from build123d import *

# Parameters (mm, degrees)
F1_DEPTH = 50


with BuildPart() as f1:
    # F0 (on Right) → F1 (new body)
    with BuildSketch(Plane.YZ):
        Polygon((40, 40), (0, 0), (4.242641, 0), (12, 7.757359), (44.242641, 40), align=None)
        Polygon((12, 7.757359), (4.242641, 0), (12, 0), align=None)
    extrude(amount=F1_DEPTH)


solid = f1.part
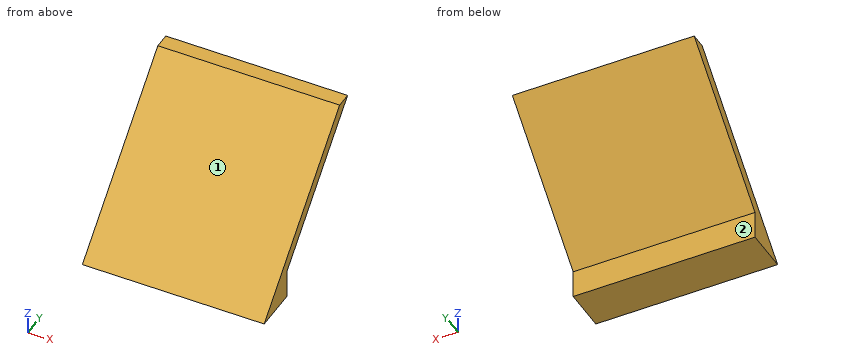
The listing builds one solid part. Answer for the finished solid, in the listing's coordinates (mm). Face numbers are marked on the shaded views. A direction names the side the tool comes from. Coordinates: 2 decimals unless noted, no trailing zeros. Loops run counter-clockwise (first coordinate to the right, second up) from the corner with the lowest first, then second, coordinate; pieces in that order, holes last. Notation, with made-up numbers: M 46.25,-1 L 61.25,-1 A30 cw 61.25,33 Z; hole C 75.5,49.5 d2. An arc over 180 degrees is marked long. Answer in a Markdown table with one row per item.
1) Given pin 1 (5 mm diameter, centred on x = 42.5, y = 35, fed in from +Z); pin 2 (1.5 mm diameter, centred on y = 22, z = 17, fed in from +X); pin 3 (2 mm diameter, centred on x = 33.5, y = 38, fed in from -Z); pin 4 (3 mm diameter, centred on x = 5, y = 15, fed in from -Z), each flat-ended and moving along its own axis, determine where each tip first touches the part or whether it passes through.
Answers below:
| item | result |
|---|---|
| pin 1 | z = 37.5 |
| pin 2 | x = 50 |
| pin 3 | z = 32.76 |
| pin 4 | z = 9.26 |
2) Find section A-A (x = 30.5). Determine the outline of the cut face in (y, z).
Answers below:
| item | result |
|---|---|
| outline | M 0,0 L 12,0 L 12,7.76 L 44.24,40 L 40,40 Z |
3) Find section C-C (z = 4.5). Determine the outline of the cut face in (x, y).
Answers below:
| item | result |
|---|---|
| outline | M 0,4.5 L 50,4.5 L 50,12 L 0,12 Z |
4) Which of the six approach directions +Z, -Z, +X, -X, +Y, -Y give full straight-line access (tool end or side, diameter ignored) to the marked faces 1 and 2?
Answers below:
| item | result |
|---|---|
| face 1 | +Z, +X, -X, -Y |
| face 2 | -Z, +X, -X, +Y |
5) Find section B-B (y = 5.5). Determine the outline of the cut face in (x, z).
Answers below:
| item | result |
|---|---|
| outline | M 0,0 L 50,0 L 50,5.5 L 0,5.5 Z |
6) Find the intervals of material crossed by probe 1 along Z at (x, y) = (39.5, 23); probe 2 along Y at (x, z) = (47.5, 15); probe 3 along Y at (x, z) = (44, 31), in increasing order.
Answers below:
| item | result |
|---|---|
| probe 1 | 18.76 to 23 |
| probe 2 | 15 to 19.24 |
| probe 3 | 31 to 35.24 |
